For this review, take the finished solid that the model builds, in its own axes (mm). A direction names the side the tool comes from. Coordinates: 2 decimals unless noted, no trailing zeros. Write each loop counter-clockwise with the first axis right and the second up, starting at its lowest first coordinate (ties: lowest second). Pieces come first, ordered by that corner, then holes.
1) We need section A-A on z = -3.5. Write out the cut boundary in (x, y).
2) For faces 1 (the face through (33.17, 0.8, -1.35)), 2 (the face through (31, -2, 0)), 3 (the face through (3.014, -0.931, -2.957)), 4 (the face through (33, -1.57, 0)), 5 (the face through (33.17, 0.77, 1.37)), list the 3-axis set-ups (+Z, -Z, +X, -X, +Y, -Y) from which the entire face can be reached by the end or side of a thin tool; tool diameter is ignored.
3) We need section D-D on z = 3.75. Write out the cut boundary in (x, y).
4) We need section B-B on x = 6.5. Write out the cut boundary in (y, z), then the cut area to 3 significant figures.
5) To check wall thickness, follow line 1 along Y through (x, z) = (5, 0); line 2 along Y through (x, z) = (3.5, 0); line 3 along X through (y, z) = (2, 3.5). State the ranges of each line that lie inside material, in increasing order.
6) Mouldability with a two-part tool opening along X and no side actions: class faces 6 (the face through (4, -1.1, -3.1)), 7 (the face through (33.17, -0.8, 1.35)), 8 (the face through (2, -1.1, 3.1)), 9 (the face through (9.12, -0.21, -0.05)) as pulls with the +X half, pulls with the -X half, needs draft (parallel to the pull), parting line crosses it, or undercut.
7) We need section C-C on x = 23.5. Write out the cut boundary in (y, z).
8) Insertion check: P1, Ø0.9, axis at x = 33, z = 0, coming from the -Y side; P2, Ø2, axis at x = 28.5, z = 2, coming from the -Y side; P3, Ø3, axis at x = 25.5, z = -3.5, coming from the -Y side. Each pin has a flat end and moves straight along its axis. Give the tip position at first contact, or say it passes through.
from build123d import *

# Parameters (mm, degrees)
SKETCH_2_W                  = 4.4
SKETCH_2_H                  = 0.93
CUT_EXTRUDE_1_DEPTH         = 36.967485317
PATTERN_CIRCULAR_1_COUNT    = 6
HOLE_WIZARD_M31_D           = 2.5
HOLE_WIZARD_M31_DEPTH       = 8.5
HOLE_WIZARD_M31_CSINK_D     = 3.2
HOLE_WIZARD_M31_CSINK_ANGLE = 90
HOLE_WIZARD_M31_TIP         = 0.751075774


with BuildPart() as part:
    # Sketch 1 → Revolve 1 (revolve)
    with BuildSketch(Plane.XY, mode=Mode.PRIVATE) as revolve_1_sk:
        Polygon((0, 0), (0, 4.5), (2, 4.5), (2, 3.1), (4, 3.1), (4, 4.5), (23, 4.5), (23, 2.5), (35.4, 2.5), (35.4, 0), align=None)
    revolve(revolve_1_sk.sketch.rotate(Axis((0, 0, 0), (-1, 0, 0)), 90), axis=Axis((0, 0, 0), (-1, 0, 0)))

    # Sketch 2 → Cut-Extrude 1 (cut, symmetric)
    with BuildSketch(Plane.XY):
        with Locations((33.2, 2.035)):
            Rectangle(SKETCH_2_W, SKETCH_2_H)
    cut_extrude_1 = extrude(amount=CUT_EXTRUDE_1_DEPTH, both=True, mode=Mode.SUBTRACT)

    # Pattern Circular 1: Cut-Extrude 1 ×6 about axis
    pattern_circular_1_axis = Axis((0, 0, 0), (1, 0, 0))
    for i in range(1, PATTERN_CIRCULAR_1_COUNT):
        add(cut_extrude_1.rotate(pattern_circular_1_axis, i * 360 / PATTERN_CIRCULAR_1_COUNT), mode=Mode.SUBTRACT)

    # Hole Wizard M31
    with Locations(Plane.ZY):
        with Locations((0, 0)):
            CounterSinkHole(HOLE_WIZARD_M31_D / 2, HOLE_WIZARD_M31_CSINK_D / 2, depth=HOLE_WIZARD_M31_DEPTH, counter_sink_angle=HOLE_WIZARD_M31_CSINK_ANGLE)
            with Locations((0, 0, -(HOLE_WIZARD_M31_DEPTH + HOLE_WIZARD_M31_TIP / 2))):  # 118° drill point
                Cone(0, HOLE_WIZARD_M31_D / 2, HOLE_WIZARD_M31_TIP, mode=Mode.SUBTRACT)


solid = part.part
Result:
1. outline: (0, -2.83) - (2, -2.83) - (2, 2.83) - (0, 2.83) - close; (4, -2.83) - (23, -2.83) - (23, 2.83) - (4, 2.83) - close
2. face 1: -Z, +X, +Y
2. face 2: +X
2. face 3: none
2. face 4: +Z, -Z, +X, -Y
2. face 5: +Z, +X, +Y
3. outline: (0, -2.49) - (2, -2.49) - (2, 2.49) - (0, 2.49) - close; (4, -2.49) - (23, -2.49) - (23, 2.49) - (4, 2.49) - close
4. outline: circle Ø9 at (0, 0); hole circle Ø2.5 at (0, 0)
4. area: 58.7 mm2
5. line 1: y = -4.5 to -1.25, 1.25 to 4.5
5. line 2: y = -3.1 to -1.25, 1.25 to 3.1
5. line 3: x = 0 to 2, 4 to 23
6. face 6: undercut
6. face 7: needs draft
6. face 8: undercut
6. face 9: pulls with the -X half
7. outline: circle Ø5 at (0, 0)
8. P1: stops at y = -1.57
8. P2: stops at y = -2.29
8. P3: stops at y = -1.5
